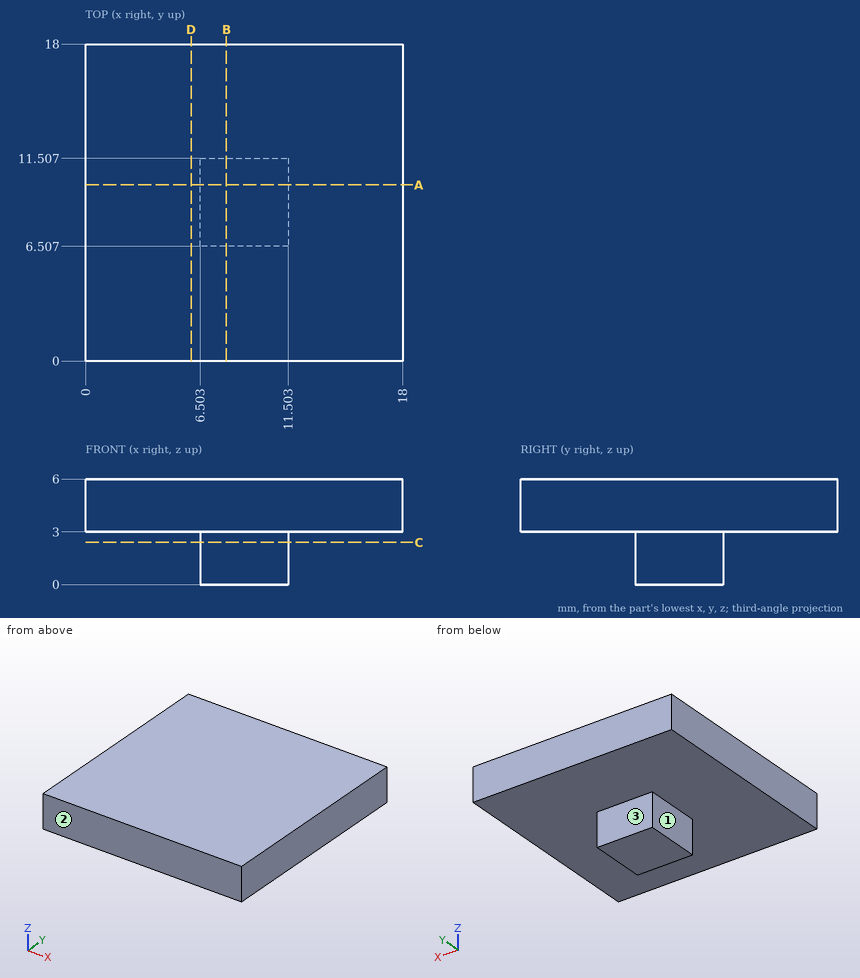
Check sheet for the drawn part. Datum: minimum x, y, z corner. Units: mm. A direction names the side the tool comes from. Coordinates: 2 decimals unless noted, no trailing zeros. Order: outer loops, then holes, each group sorted by start corner. A loop starts at its lowest first (then second) coordinate and runs counter-clockwise, first axis right, second up. Notation, with made-up numbers: M -38.75,83 L -15.75,83 A20 ccw -15.75,96 Z; hole C 34.25,80.25 d11. An arc over 180 degrees is marked long. One line per item, written item: value. Start each with the question number.
Item 1: Sectioned sample at C-C (z = 2.4). Enter the section's corners in (x, y).
Item 2: Sectioned sample at D-D (x = 6). Enter the section's corners in (y, z), then the cut area to 3 significant figures.
Item 3: Gauge pin test, flat ends, axial feed: pin 1 (1.5 mm diameter, centred on x = 9, z = 1, fed in from +Y); pin 2 (1.5 mm diameter, centred on y = 10, z = 2, fed in from -X); pin 3 (0.9 mm diameter, centred on y = 8.5, z = 1.5, fed in from +X). Record the tip position at first contact, or that the pin passes through.
Item 4: Sectioned sample at A-A (y = 10). Enter the section's corners in (x, z), then the cut area to 3 significant figures.
Item 5: Sectioned sample at B-B (x = 8). Enter the section's corners in (y, z).
Item 6: Scan lines: probe 1 along Z at (x, y) = (8.5, 17.25); probe 2 along Y at (x, z) = (10, 1.6); probe 3 along X at (y, z) = (10.75, 2.6). Record each from-to range of solid material in increasing order.
Item 7: Access from +Z, -Z, +X, -X, +Y, -Y to the whole of each face (thin tool, end or side, straight path). Record for the marked faces 1, 2 and 3.
Conclusion:
1. outline: M 6.5,6.51 L 11.5,6.51 L 11.5,11.51 L 6.5,11.51 Z
2. outline: M 0,3 L 18,3 L 18,6 L 0,6 Z
2. area: 54.0 mm^2
3. pin 1: stops at y = 11.51
3. pin 2: stops at x = 6.5
3. pin 3: stops at x = 11.5
4. outline: M 0,3 L 6.5,3 L 6.5,0 L 11.5,0 L 11.5,3 L 18,3 L 18,6 L 0,6 Z
4. area: 69.0 mm^2
5. outline: M 0,3 L 6.51,3 L 6.51,0 L 11.51,0 L 11.51,3 L 18,3 L 18,6 L 0,6 Z
6. probe 1: z = 3 to 6
6. probe 2: y = 6.51 to 11.51
6. probe 3: x = 6.5 to 11.5
7. face 1: -Z, -X, +Y, -Y
7. face 2: +Z, -Z, +X, -X, -Y
7. face 3: -Z, +X, -X, +Y
